```python
from build123d import *

# Parameters (mm, degrees)
F0_W      = 100
F0_H      = 30
F1_DEPTH  = 71.1
F2_R      = 12.0710678119
F3_R      = 14.4852813742
F4_R      = 16.3433184156
F5_DEPTH  = 14.5
F6_R      = 11.1772790222
F7_DEPTH  = 5.8
F8_R      = 11.70616328
F9_DEPTH  = 7.2
F10_DEPTH = 30.1
F11_DEPTH = 25
F12_DEPTH = 25
F13_DEPTH = 5
F15_DEPTH = 1.2


with BuildPart() as f1:
    # F0 (on Top) → F1 (new body)
    with BuildSketch(Plane.XY):
        with Locations((-23.7509091896, -13.5745047592)):
            Rectangle(F0_W, F0_H)
    extrude(amount=F1_DEPTH)

    # F2
    f2_edges = [f1.edges().sort_by_distance(p)[0] for p in [
        (-23.750909, -28.574505, 71.1),
    ]]
    fillet(f2_edges, radius=F2_R)

    # F3
    f3_edges = [f1.edges().sort_by_distance(p)[0] for p in [
        (-23.750909, 1.425495, 71.1),
    ]]
    fillet(f3_edges, radius=F3_R)

    # F4 (on face) → F5 (join)
    with BuildSketch(Plane.XZ.offset(28.5745047592)):
        with Locations((-48.9764623344, 24.0149181336)):
            Circle(F4_R)
    extrude(amount=F5_DEPTH)

    # F6 (on face) → F7 (join)
    with BuildSketch(Plane.XZ.offset(43.0745047592)):
        with Locations((-48.9764623344, 24.0149181336)):
            Circle(F6_R)
    extrude(amount=-F7_DEPTH)

    # F8 (on face) → F9 (join)
    with BuildSketch(Plane.XZ.offset(43.0745047592)):
        with Locations((-48.9764623344, 24.0149181336)):
            Circle(F8_R)
    extrude(amount=F9_DEPTH)

    # F10 (cut): a face of the model
    f10_faces = [f1.faces().sort_by_distance(p)[0] for p in [
        (-48.9764623344, -50.2745047592, 24.0149181336),
    ]]
    extrude(f10_faces, amount=-F10_DEPTH, mode=Mode.SUBTRACT)

    # F11 (add): a face of the model
    f11_faces = [f1.faces().sort_by_distance(p)[0] for p in [
        (-19.5707016042, -28.5745047592, 30.4258138837),
    ]]
    extrude(f11_faces, amount=F11_DEPTH)

    # F12 (cut): a face of the model
    f12_faces = [f1.faces().sort_by_distance(p)[0] for p in [
        (-19.5707016042, -53.5745047592, 30.4258138837),
    ]]
    extrude(f12_faces, amount=-F12_DEPTH, mode=Mode.SUBTRACT)

    # F13 (cut): a face of the model
    f13_faces = [f1.faces().sort_by_distance(p)[0] for p in [
        (-64.8575218988, -43.0745047592, 24.0149181336),
    ]]
    extrude(f13_faces, amount=-F13_DEPTH, mode=Mode.SUBTRACT)

    # F14 (on face) → F15 (join)
    with BuildSketch(Plane.XY.offset(71.1)):
        with BuildLine():
            ThreePointArc((5.4310929405, -16.5034369473), (6.3738933306, -14.8950718744), (6.7016692178, -13.0597861334))
            Line((6.7016692178, -13.0597861334), (-3.9022553523, -13.0597861334))
            ThreePointArc((-3.9022553523, -13.0597861334), (-3.5744794652, -14.8950718744), (-2.6316790751, -16.5034369473))
            Line((-2.6316790751, -16.5034369473), (5.4310929405, -16.5034369473))
        make_face()
        with BuildLine():
            Line((-3.9022553523, -13.0597861334), (6.7016692178, -13.0597861334))
            ThreePointArc((6.7016692178, -13.0597861334), (1.3997069327, -7.7578238484), (-3.9022553523, -13.0597861334))
        make_face()
        with BuildLine():
            ThreePointArc((-2.6316790751, -16.5034369473), (1.3997069327, -18.3617484184), (5.4310929405, -16.5034369473))
            Line((5.4310929405, -16.5034369473), (-2.6316790751, -16.5034369473))
        make_face()
    extrude(amount=F15_DEPTH)


solid = f1.part
```
Could you check a few things on this model? Use its own coordinates, in mm. A direction names the side the tool comes from. Round coordinates to 2 decimals unless told otherwise and drop trailing zeros. Loops run counter-clockwise (first coordinate to the right, second up) from the corner with the lowest first, then second, coordinate; pieces in that order, holes last. Notation, with made-up numbers: (86.25, -18.75) -> (126.25, -18.75) arc R25 cw to (126.25, 4.25) -> close; hole circle Ø7 at (-36, 0.25). An arc over 180 degrees is marked (long way). Put each result on its own line as item: value.
Q1. I want a section at A-A on y = -10. Write out the boundary of the cut face in (x, z), and give its area (3 significant figures).
Checks:
outline: (-73.75, 0) -> (26.25, 0) -> (26.25, 70.77) -> (-73.75, 70.77) -> close; (-2.93, 71.1) -> (5.73, 71.1) -> (5.73, 72.3) -> (-2.93, 72.3) -> close
area: 7,090 mm2
Q2. I want a section at C-C on y = -22. Write out the boundary of the cut face in (x, z), and give its area (3 significant figures).
Checks:
outline: (-73.75, 0) -> (26.25, 0) -> (26.25, 69.78) -> (-73.75, 69.78) -> close; hole circle Ø23.41 at (-48.98, 24.01)
area: 6,550 mm2
Q3. Thinking about a two-plate mould opening in Z: for faces 4 (the flat face through (16, -15, 71.1)), 5 (the cylindrical face through (-57.6, -29.25, 31.93)), 6 (the flat face through (-73.751, -13, 35)), which applies, pulls with the +Z half, pulls with the -Z half, needs draft (parallel to the pull), parting line crosses it, or undercut?
Checks:
face 4: pulls with the +Z half
face 5: undercut
face 6: needs draft
Q4. Please list where these lines run through material, in increasing order: line 1 (Z direction, x = 20, y = -13); line 2 (Y direction, x = -57, z = 17.5); line 3 (X direction, y = -26, z = 23). Write a range as from..to.
Checks:
line 1: 0..71.1
line 2: -20.17..1.43
line 3: -73.75..-60.64, -37.31..26.25
Q5. For pin 1 Ø21 at (x, z) = (-48.98, 24.01) entering from -Y; pin 2 Ø4 at (x, y) = (20, -15) entering from +Z; pin 3 Ø2 at (x, y) = (6, -24.5) entering from +Z, each with a flat end and sliding along its axis, tell me the tip position at first contact or that it passes through.
Checks:
pin 1: y = -20.17
pin 2: z = 71.1
pin 3: z = 68.87
Q6. Which directions (+Z, -Z, +X, -X, +Y, -Y) give clear straight access to the entire face, cutting with the end or side of a thin tool? Please do faces 1 (the cylindrical face through (-65.304, -33.391, 24.734)), 2 (the flat face through (-24, -13, 0)), 3 (the flat face through (1.33, -10.96, 71.1)).
Checks:
face 1: -Y
face 2: -Z, +X, -X, +Y, -Y
face 3: none
Q7. I want a section at D-D on z = 20. Write out the boundary of the cut face in (x, y).
Checks:
outline: (-73.75, -28.57) -> (-64.82, -28.57) -> (-64.82, -38.07) -> (-59.97, -38.07) -> (-59.97, -20.17) -> (-37.98, -20.17) -> (-37.98, -38.07) -> (-33.13, -38.07) -> (-33.13, -28.57) -> (26.25, -28.57) -> (26.25, 1.43) -> (-73.75, 1.43) -> close
Q8. I want a section at B-B on x = -10. Write out the boundary of the cut face in (y, z), and give its area (3 significant figures).
Checks:
outline: (-28.57, 0) -> (1.43, 0) -> (1.43, 56.61) arc R14.49 ccw to (-13.06, 71.1) -> (-16.5, 71.1) arc R12.07 ccw to (-28.57, 59.03) -> close
area: 2,060 mm2
